from build123d import *

# Parameters (mm, degrees)
SKETCH2_W               = 5
SKETCH2_H               = 74.664160083
SKETCH2_W_2             = 10
SKETCH2_H_2             = 5
SKETCH2_R               = 1.15
BOSS_EXTRUDE1_DEPTH     = 1.5
SKETCH3_W               = 13
SKETCH3_H               = 74.664160083
BOSS_EXTRUDE2_DEPTH     = 1
SKETCH5_W               = 97.96
SKETCH5_H               = 74.648794292
BOSS_EXTRUDE3_DEPTH     = 1
SKETCH6_R               = 25
SKETCH6_R_2             = 23
BOSS_EXTRUDE4_DEPTH     = 18
SKETCH8_R               = 27.5
SKETCH8_R_2             = 23.5
BOSS_EXTRUDE6_DEPTH     = 2.5
SKETCH13_W              = 18
SKETCH13_H              = 23
BOSS_EXTRUDE7_DEPTH     = 1
SKETCH15_R              = 3.75
CUT_EXTRUDE3_DEPTH      = 1
BODY_MOVE_COPY2_ANGLE   = 90
SKETCH16_R              = 3.75
BOSS_EXTRUDE8_DEPTH     = 6
SKETCH17_R              = 0.9
CUT_EXTRUDE4_DEPTH      = 46
CUT_EXTRUDE4_DEPTH_BACK = 44
SKETCH18_W              = 142.524598678
SKETCH18_H              = 112.115255427
CUT_EXTRUDE5_DEPTH      = 7
SKETCH20_R              = 32
BOSS_EXTRUDE9_DEPTH     = 3
SKETCH23_W              = 15
SKETCH23_H              = 15
BOSS_EXTRUDE11_DEPTH    = 65


with BuildPart() as part:
    # Sketch2 → Boss-Extrude1 (new body)
    with BuildSketch(Plane.XY):
        with Locations((376.369557123, 140.674264472)):
            Rectangle(SKETCH2_W, SKETCH2_H)
        with Locations((368.869557123, 175.506344513)):
            Rectangle(SKETCH2_W_2, SKETCH2_H_2)
        with Locations((366.369557123, 175.506344513)):
            Circle(SKETCH2_R, mode=Mode.SUBTRACT)
        with Locations((368.869557123, 105.84218443)):
            Rectangle(SKETCH2_W_2, SKETCH2_H_2)
        with Locations((366.369557123, 105.84218443)):
            Circle(SKETCH2_R, mode=Mode.SUBTRACT)
    boss_extrude1 = extrude(amount=BOSS_EXTRUDE1_DEPTH)

    # Sketch3 → Boss-Extrude2 (add)
    with BuildSketch(Plane(origin=(378.869557123, 0, 0), x_dir=(0, 0, -1), z_dir=(1, 0, 0))):
        with Locations((5, 140.674264472)):
            Rectangle(SKETCH3_W, SKETCH3_H)
    extrude(amount=BOSS_EXTRUDE2_DEPTH)

    # Mirror3: Boss-Extrude1 across plane
    add(boss_extrude1.mirror(Plane(origin=(0, 0, -5), x_dir=(1, 0, 0), z_dir=(0, 0, -1))))


with BuildPart() as body_2:
    # Body-Move/Copy1: copy of part
    add(part.part.moved(Location((0, 0, 84.96))))


with BuildPart() as part_1:
    add(part.part)

    add(body_2.part)  # Boss-Extrude3 merges body 2
    # Sketch5 → Boss-Extrude3 (add)
    with BuildSketch(Plane(origin=(379.869557123, 0, 0), x_dir=(0, 0, -1), z_dir=(1, 0, 0))):
        with Locations((-37.48, 140.681947367)):
            Rectangle(SKETCH5_W, SKETCH5_H)
    extrude(amount=-BOSS_EXTRUDE3_DEPTH)

    # Sketch6 → Boss-Extrude4 (add)
    with BuildSketch(Plane.ZY.offset(-378.869557123)):
        with Locations(Location((37.48, 140.674264472, 0), (0, 0, 270))):
            Circle(SKETCH6_R)
        with Locations(Location((37.48, 140.674264472, 0), (0, 0, 270))):
            Circle(SKETCH6_R_2, mode=Mode.SUBTRACT)
    extrude(amount=BOSS_EXTRUDE4_DEPTH)

    # Sketch8 → Boss-Extrude6 (add)
    with BuildSketch(Plane.ZY.offset(-360.869557123)):
        with Locations(Location((37.48, 140.674264472, 0), (0, 0, 270))):
            Circle(SKETCH8_R)
        with Locations(Location((37.48, 140.674264472, 0), (0, 0, 270))):
            Circle(SKETCH8_R_2, mode=Mode.SUBTRACT)
    extrude(amount=BOSS_EXTRUDE6_DEPTH)

    # Sketch13 → Boss-Extrude7 (add)
    with BuildSketch(Plane.ZY.offset(-378.869557123)):
        with Locations((37.48, 189.506344513)):
            Rectangle(SKETCH13_W, SKETCH13_H)
        with Locations((37.48, 91.857550221)):
            Rectangle(SKETCH13_W, SKETCH13_H)
    extrude(amount=-BOSS_EXTRUDE7_DEPTH)

    # Sketch15 → Cut-Extrude3 (cut)
    with BuildSketch(Plane.ZY.offset(-378.869557123)):
        with Locations(Location((37.48, 195.006344513, 0), (0, 0, 270))):
            Circle(SKETCH15_R)
        with Locations(Location((37.48, 86.357550221, 0), (0, 0, 270))):
            Circle(SKETCH15_R)
    extrude(amount=-CUT_EXTRUDE3_DEPTH, mode=Mode.SUBTRACT)


with BuildPart() as part_2:
    # Body-Move/Copy2: moved
    add(part_1.part.rotate(Axis((371.869557123, 140.681947367, 0), (0, 0, 1)), BODY_MOVE_COPY2_ANGLE))

    # Sketch16 → Boss-Extrude8 (add)
    with BuildSketch(Plane(origin=(0, 148.681947367, 0), x_dir=(1, 0, 0), z_dir=(0, 1, 0))):
        Polygon((334.545159977, -28.48), (334.545159977, 11.5), (409.20932006, 11.5), (409.193954269, -28.48), (432.193954269, -28.48), (432.193954269, -46.48), (409.193954269, -46.48), (409.20932006, -86.46), (334.545159977, -86.46), (334.545159977, -46.48), (311.545159977, -46.48), (311.545159977, -28.48), align=None)
        with Locations((317.545159977, -37.48)):
            Circle(SKETCH16_R, mode=Mode.SUBTRACT)
        with Locations((426.193954269, -37.48)):
            Circle(SKETCH16_R, mode=Mode.SUBTRACT)
    extrude(amount=BOSS_EXTRUDE8_DEPTH)

    # Sketch17 → Cut-Extrude4 (cut, two sides)
    with BuildSketch(Plane.XY.offset(37.48)) as cut_extrude4_sk:
        with Locations(Location((371.877240018, 135.181947367, 0), (0, 0, 180))):
            Circle(SKETCH17_R)
    extrude(amount=CUT_EXTRUDE4_DEPTH, mode=Mode.SUBTRACT)
    extrude(cut_extrude4_sk.sketch, amount=-CUT_EXTRUDE4_DEPTH_BACK, mode=Mode.SUBTRACT)

    # Sketch18 → Cut-Extrude5 (cut)
    with BuildSketch(Plane(origin=(0, 154.681947367, 0), x_dir=(1, 0, 0), z_dir=(0, 1, 0))):
        with Locations((368.644323748, -41.089189729)):
            Rectangle(SKETCH18_W, SKETCH18_H)
    extrude(amount=-CUT_EXTRUDE5_DEPTH, mode=Mode.SUBTRACT)


with BuildPart() as body_2_2:
    # of the pieces the cut leaves, the one that is kept (cut_extrude5_keep)
    add(part_2.part.solids().sort_by_distance((396.877240018, 147.681947367, 37.48))[0])

    # Sketch20 → Boss-Extrude9 (add)
    with BuildSketch(Plane(origin=(0, 147.681947367, 0), x_dir=(1, 0, 0), z_dir=(0, 1, 0))):
        with Locations(Location((371.877240018, -37.48, 0), (0, 0, 180))):
            Circle(SKETCH20_R)
    extrude(amount=BOSS_EXTRUDE9_DEPTH)

    # Sketch23 → Boss-Extrude11 (add)
    with BuildSketch(Plane(origin=(0, 150.681947367, 0), x_dir=(1, 0, 0), z_dir=(0, 1, 0))):
        with Locations((371.877240018, -37.48)):
            Rectangle(SKETCH23_W, SKETCH23_H)
    extrude(amount=BOSS_EXTRUDE11_DEPTH)


solid = body_2_2.part
Check sheet for the modelled part. Datum: model origin and axes. Units: mm. A direction names the side the tool comes from. Round coordinates to 2 decimals unless told otherwise and drop trailing zeros. Order: outer loops, then holes, each group sorted by start corner. A loop starts at its lowest first (then second) coordinate and runs counter-clockwise, first axis right, second up. Notation, with made-up numbers: M 55.5,71 L 99.5,71 A18 ccw 99.5,93 Z; hole C 62,56.5 d8. An arc over 180 degrees is marked long. One line per item, written item: value. Start each with the question number.
1. Section check B-B on y = 184. Enter the section's corners in (x, z).
2. Section check A-A on z = 37.48. Enter the section's corners in (x, y), and give its area (3 significant figures).
3. Scan lines: line 1 along Y through (x, z) = (382, 63); line 2 along Y through (x, z) = (395, 28.5); line 3 along Y through (x, z) = (358.5, 47). Record each from-to range of solid material in increasing order.
4. Section check C-C on x = 387. Enter the section's corners in (y, z).
5. Release check for a two-part mould opening along Z. For faces 4 (the flat face through (378, 129.682, 13)), 5 (the cylindrical face through (344.404, 128.449, 38.689)), 6 (the cylindrical face through (393.123, 138.808, 28.671)) record: released by +Z, released by -Z, zero draft, split by the parting line, or undercut.
6. Gauge pin test, flat ends, axial feed: P1, Ø3, axis at y = 157.5, z = 33.5, coming from the +X side; P2, Ø2.5, axis at x = 371.88, y = 135.18, coming from the -Z side; P3, Ø12, axis at y = 178.5, z = 53, coming from the -X side; P4, Ø4, axis at x = 397.5, z = 19.5, coming from the +Y side. Record the tip position at first contact, or that the pin passes through.
7. Access from +Z, -Z, +X, -X, +Y, -Y to the whole of each face (thin tool, end or side, straight path). Record for faces 1 (the flat face through (379.377, 183, 38)), 2 (the cylindrical face through (348.4, 128.4, 38.5)), 3 (the cylindrical face through (346.9, 138.81, 38.58)).
8. Section check D-D on z = 50.5. Enter the section's corners in (x, y), and give its area (3 significant figures).
Results found:
1. outline: M 364.38,29.98 L 379.38,29.98 L 379.38,44.98 L 364.38,44.98 Z
2. outline: M 339.88,147.68 L 346.88,147.68 L 346.88,129.68 L 344.38,129.68 L 344.38,127.18 L 348.38,127.18 L 348.38,129.68 L 348.88,129.68 L 348.88,147.68 L 394.88,147.68 L 394.88,129.68 L 395.38,129.68 L 395.38,127.18 L 399.38,127.18 L 399.38,129.68 L 396.88,129.68 L 396.88,147.68 L 403.88,147.68 L 403.88,150.68 L 379.38,150.68 L 379.38,215.68 L 364.38,215.68 L 364.38,150.68 L 339.88,150.68 Z
2. area: 1,260 mm^2
3. line 1: 127.18 to 129.68, 147.68 to 150.68
3. line 2: 127.18 to 150.68
3. line 3: 147.68 to 150.68
4. outline: M 127.18,14.51 L 129.68,14.51 L 129.68,17.57 L 147.68,17.57 L 147.68,9.28 L 150.68,9.28 L 150.68,65.68 L 147.68,65.68 L 147.68,57.39 L 129.68,57.39 L 129.68,60.45 L 127.18,60.45 L 127.18,55.47 L 129.68,55.47 L 129.68,54.81 L 147.68,54.81 L 147.68,20.15 L 129.68,20.15 L 129.68,19.49 L 127.18,19.49 Z
5. face 4: zero draft
5. face 5: split by the parting line
5. face 6: undercut
6. P1: x = 379.38
6. P2: z = 12.48
6. P3: through
6. P4: y = 150.68
7. face 1: +Z, -Z, +X, +Y
7. face 2: -Y
7. face 3: none
8. outline: M 342.65,147.68 L 350.54,147.68 L 350.54,129.68 L 347.65,129.68 L 347.65,127.18 L 352.31,127.18 L 352.31,129.68 L 352.92,129.68 L 352.92,147.68 L 390.84,147.68 L 390.84,129.68 L 391.44,129.68 L 391.44,127.18 L 396.1,127.18 L 396.1,129.68 L 393.22,129.68 L 393.22,147.68 L 401.11,147.68 L 401.11,150.68 L 342.65,150.68 Z
8. area: 284 mm^2
